Input: dimensioned drawing with shaded views. Units: mm. Origin: part minimum x, y, z. A direction names the side the tool comes from. Coordinates: 2 decimals unless noted, no trailing zeros. Loops run counter-clockwise (first coordinate to the right, second up) from the corner with the lowest first, then second, coordinate; pieces in that order, holes last. Notation, with made-up numbers: (-34.5, 37) - (-3.5, 37) arc R13 cw to (-3.5, 42) - close; hole circle Ø6 at (38, 5.25). An arc over 180 degrees is marked (long way). Write item = value, one per line. Start each with the question number.
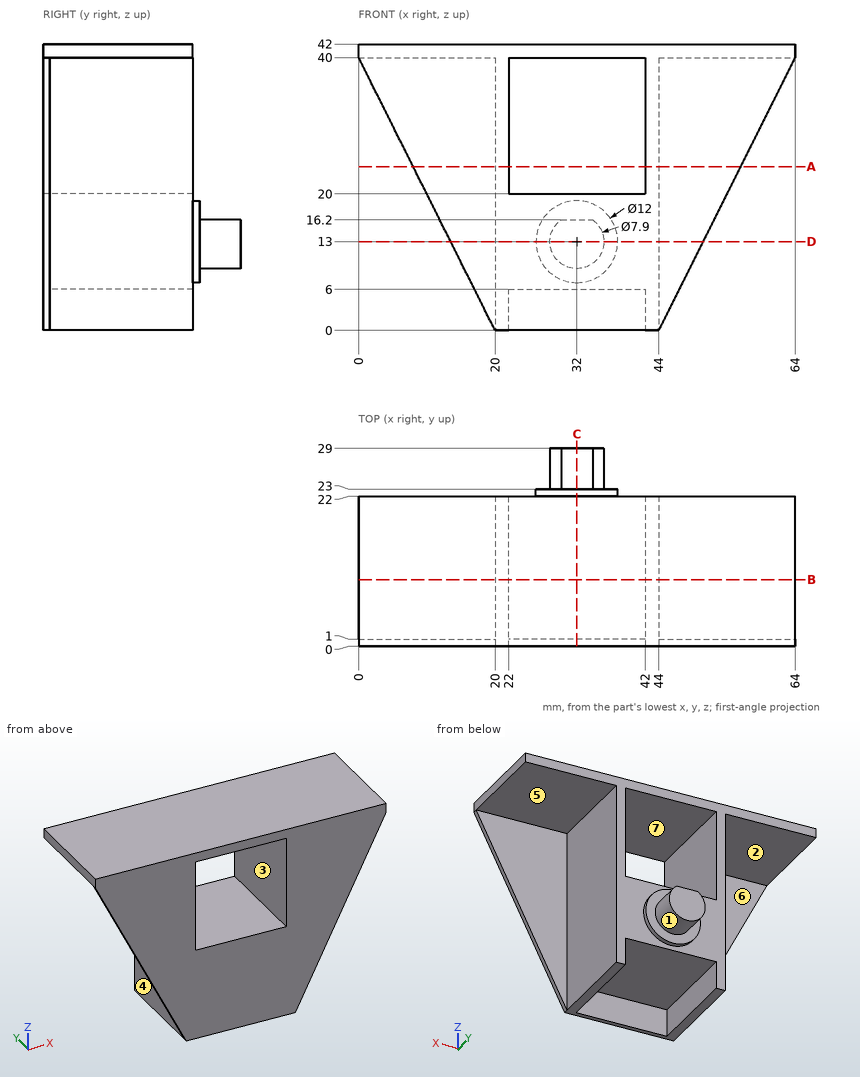
Item 1: Access query for the marked faces 5, 6 and 7. Directions: +Z, -Z, +X, -X, +Y, -Y. A direction counts if a zero-diameter tool reaches every point of the face in a straight line with its end or side. Return the directions, or none.
Item 2: Cut plane B-B on y = 9.75. Return loops of the section in (x, z), plus the area to 3 significant figures.
Item 3: Pull-direction query (X, two-part tool) for the marked faces 1, 2, 3 and 4; classes: pulls with the +X half, pulls with the -X half, needs draft (parallel to the pull), parting line crosses it, or undercut.
Item 4: Cut plane D-D on z = 13. Return loops of the section in (x, y), plus the area to 3 significant figures.
Item 5: Ray query, line 1 (X direction, y = 17.5, z = 20.5); line 2 (Z direction, x = 32.5, y = 17.5); line 3 (Y direction, x = 54, z = 25). Return the intervals inside material, ascending.
Item 6: Cut plane A-A on z = 24. Return loops of the section in (x, y), plus the area to 3 significant figures.
Item 7: Cut plane C-C on x = 32. Return loops of the section in (y, z).
Item 8: Pin query (flat end, axial travel): pin 1 (16 mm diameter, centred on x = 10, y = 15, fed in from -Z); pin 2 (17 mm diameter, centred on y = 11.5, z = 12.5, fed in from +X); pin 3 (1 mm diameter, centred on y = 20.5, z = 32, fed in from -X). Return the tip coordinate at first contact, or that it passes through.
Recorded:
q1.face_5 = -Z, +X, +Y
q1.face_6 = -Z, -X, +Y
q1.face_7 = +Y, -Y
q2.outline = (0, 40) - (20, 40) - (20, 0) - (22, 0) - (22, 6) - (42, 6) - (42, 0) - (44, 0) - (44, 40) - (64, 40) - (64, 42) - (0, 42) - close; hole (22, 20) - (42, 20) - (42, 40) - (22, 40) - close
q2.area = 568 mm²
q3.face_1 = parting line crosses it
q3.face_2 = needs draft
q3.face_3 = undercut
q3.face_4 = pulls with the -X half
q4.outline = (13.5, 0) - (50.5, 0) - (50.5, 1) - (44, 1) - (44, 22) - (38, 22) - (38, 23) - (35.95, 23) - (35.95, 29) - (28.05, 29) - (28.05, 23) - (26, 23) - (26, 22) - (20, 22) - (20, 1) - (13.5, 1) - close
q4.area = 600 mm²
q5.line_1 = 20 to 22, 42 to 44
q5.line_2 = 6 to 20, 40 to 42
q5.line_3 = 0 to 1
q6.outline = (8, 0) - (22, 0) - (22, 22) - (20, 22) - (20, 1) - (8, 1) - close; (42, 0) - (56, 0) - (56, 1) - (44, 1) - (44, 22) - (42, 22) - close
q6.area = 112 mm²
q7.outline = (0, 0) - (1, 0) - (1, 6) - (22, 6) - (22, 7) - (23, 7) - (23, 9.05) - (29, 9.05) - (29, 16.2) - (23, 16.2) - (23, 19) - (22, 19) - (22, 20) - (0, 20) - close; (0, 40) - (22, 40) - (22, 42) - (0, 42) - close
q8.pin_1 = 40
q8.pin_2 = 44
q8.pin_3 = 20
